The listing builds one solid part. Answer for the finished solid, in the listing's coordinates (mm). Face numbers are marked on the shaded views. A direction names the side the tool comes from. Coordinates: 2 decimals unless noted, no trailing zeros. Write each loop counter-clockwise with the first axis right and the second up, starting at its lowest first coordinate (ties: lowest second). Pieces come first, ordered by that corner, then holes.
(1) Which of the six approach directions +Z, -Z, +X, -X, +Y, -Y give full straight-line access (tool end or side, diameter ignored) to the marked faces 1 and 2?
(2) Given P1, Ø12, axis at y = 108, z = -11.5, coming from the +X side; P2, Ø6, axis at x = -21.5, z = 20, coming from the +Y side, each flat-ended and moving along its own axis, determine where each tip first touches the part or whether it passes through.
(3) The part is cut by section A-A on z = -26.5. Determine the outline of the cut face in (x, y).
(4) The part is cut by section C-C on y = 36.5. Determine the outline of the cut face in (x, z).
(5) The part is cut by section B-B on x = 8. Determine the outline of the cut face in (y, z).
(6) Straight lines are drawn through the part: line 1 (X direction, y = 92, z = -7); line 2 (Y direction, x = -19, z = -24). For each, find the intervals that lie inside material, in ascending order.
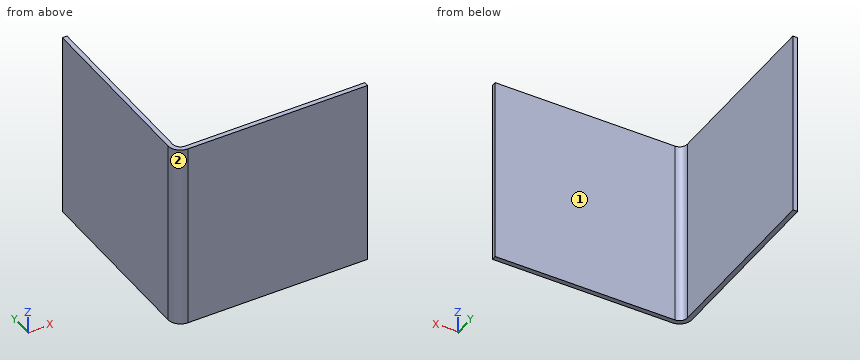
from build123d import *

# Parameters (mm, degrees)
SKETCH1_W              = 120
SKETCH1_H              = 120
BOSS_EXTRUDE1_DEPTH    = 3
SKETCH2_W              = 3
SKETCH2_H              = 120
BOSS_EXTRUDE2_DEPTH    = 123
CONVERT_SOLID2_START   = -60
CONVERT_SOLID2_DEPTH   = 120
CONVERT_SOLID2_2_DEPTH = 120


# Read off the part's stored shape, not the designer's step: Convert-Solid2
with BuildPart() as part:
    # Sketch1 → Boss-Extrude1 (new body)
    with BuildSketch(Plane(origin=(0, 0, 0), x_dir=(1, 0, 0), z_dir=(0, 1, 0))):
        Rectangle(SKETCH1_W, SKETCH1_H)
    extrude(amount=BOSS_EXTRUDE1_DEPTH)

    # Sketch2 → Boss-Extrude2 (add)
    with BuildSketch(Plane.XZ):
        with Locations((-61.5, 0)):
            Rectangle(SKETCH2_W, SKETCH2_H)
    extrude(amount=-BOSS_EXTRUDE2_DEPTH)

    # Convert-Solid2 outline → Convert-Solid2 (cut)
    with BuildSketch(Plane.XY.offset(CONVERT_SOLID2_START)):
        with BuildLine():
            Line((-63, 0), (-55, 0))
            ThreePointArc((-55, 0), (-60.656854249, 2.343145751), (-63, 8))
            Line((-63, 8), (-63, 0))
        make_face()
    extrude(amount=CONVERT_SOLID2_DEPTH, mode=Mode.SUBTRACT)

    # Convert-Solid2 2 outline → Convert-Solid2 2 (add)
    with BuildSketch(Plane.XY.offset(CONVERT_SOLID2_START)):
        with BuildLine():
            Line((-60, 3), (-55, 3))
            ThreePointArc((-55, 3), (-58.535533906, 4.464466094), (-60, 8))
            Line((-60, 8), (-60, 3))
        make_face()
    extrude(amount=CONVERT_SOLID2_2_DEPTH)


solid = part.part
Model answer:
1. face 1: +Z, -Z, +X, +Y
1. face 2: +Z, -Z, -X, -Y
2. P1: stops at x = -60
2. P2: stops at y = 3
3. outline: (-63, 8) arc R8 ccw to (-55, 0) - (60, 0) - (60, 3) - (-55, 3) arc R5 cw to (-60, 8) - (-60, 123) - (-63, 123) - close
4. outline: (-63, -60) - (-60, -60) - (-60, 60) - (-63, 60) - close
5. outline: (0, -60) - (3, -60) - (3, 60) - (0, 60) - close
6. line 1: x = -63 to -60
6. line 2: y = 0 to 3
